Here's the drawing with two shaded views (mm, measured from the low corner). I have some questions. Give positions to 0.01 mm unless a question says otherwise; leave off trailing zeros. Write each loop counter-clockwise with the first axis right and the second up, starting at its lowest first coordinate (ties: lowest second). Pieces come first, ordered by that corner, then holes. Notation, with made-up numbers: M -5.75,-19.5 L 42.25,-19.5 A16 cw 42.25,-8.5 Z; hole C 14,-13 d4. An arc over 180 degrees is marked long. Answer as a JSON object with one key per item and string values. Group by question number.
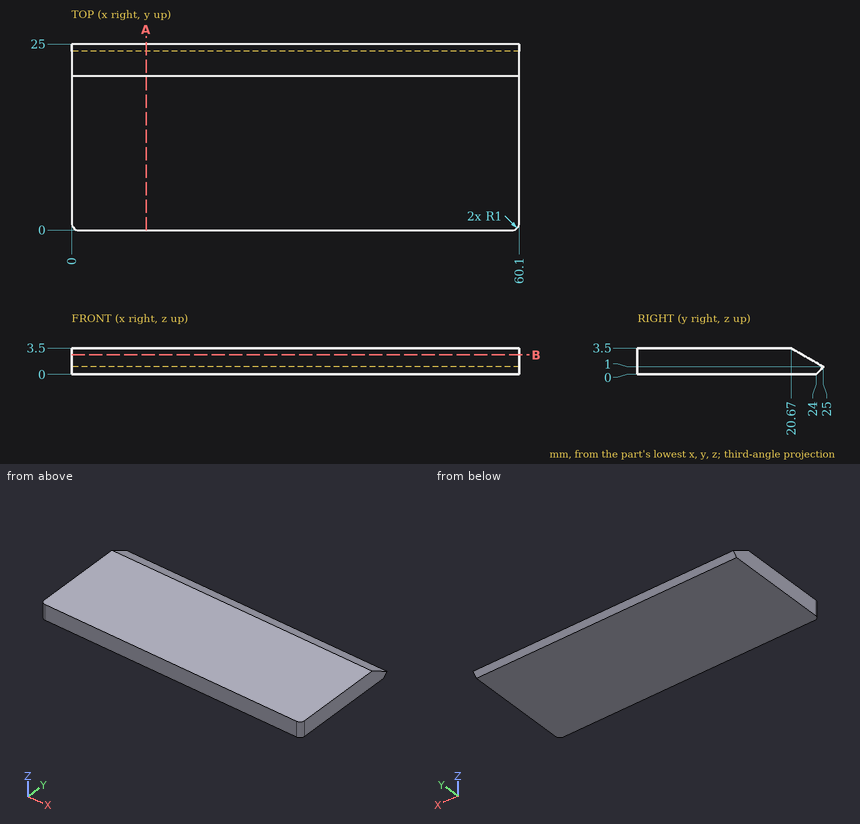
1) Please list where these lines run through material, in increasing order: line 1 along Y through (x, z) = (28.5, 2.1) (1 decimal); line 2 along Y through (x, z) = (11.5, 1.95) (1 decimal); line 3 along Z through (x, y) = (21, 23.5). Write a range as from..to.
2) If we section it at A-A, the plane x = 10: List the corners of the cut face in (y, z) for me, plus the area to 3 significant figures.
3) If we section it at B-B, the plane z = 2.6: List the corners of the cut face in (x, y) for me.
Taken from the geometry:
{
 "1": {"line 1": "0..23.1", "line 2": "0..23.4", "line 3": "0..1.87"},
 "2": {"outline": "M 0,0 L 24,0 L 25,1 L 20.67,3.5 L 0,3.5 Z", "area": "81.6 mm²"},
 "3": {"outline": "M 0,1 A1 ccw 1,0 L 59.1,0 A1 ccw 60.1,1 L 60.1,22.23 L 0,22.23 Z"}
}
